```python
from build123d import *

# Parameters (mm, degrees)
BOSS_EXTRUDE1_DEPTH = 30
SHELL1_T            = 3


with BuildPart() as part:
    # Sketch1 → Boss-Extrude1 (new body)
    with BuildSketch(Plane(origin=(0, 0, 0), x_dir=(1, 0, 0), z_dir=(0, 1, 0))):
        Polygon((20.5, 48.994047619), (-20.5, 48.994047619), (-20.5, -1.005952381), (-50, -1.005952381), (-50, -51.005952381), (50, -51.005952381), (50, -1.005952381), (20.5, -1.005952381), align=None)
    extrude(amount=BOSS_EXTRUDE1_DEPTH)

    # Shell1
    shell1_openings = [part.faces().sort_by_distance(p)[0] for p in [
        (0, 30, 11.466945289),
    ]]
    offset(amount=SHELL1_T, openings=shell1_openings, kind=Kind.INTERSECTION)


solid = part.part
```
The model under review builds one solid part; all positions refer to its coordinate system, in mm. A direction names the side the tool comes from. Coordinates: 2 decimals unless noted, no trailing zeros. Write each loop counter-clockwise with the first axis right and the second up, starting at its lowest first coordinate (ties: lowest second). Pieces come first, ordered by that corner, then holes.
1) We need section B-B on x = -17. State the section outline as (y, z) points.
2) Machinability: for faces 1 (the face through (-50, 15, 26)), 2 (the face through (23.5, 13, -27)), 3 (the face through (-38, 13, -1.994)), which of the approach directions +Z, -Z, +X, -X, +Y, -Y give a long, thin tool a straight path to every point of the face, cutting with its end or side? Answer none if there is none.
3) We need section A-A on y = 6. State the section outline as (x, z) points, then the cut area to 3 significant figures.
4) To check wall thickness, follow probe 1 along X at (y, z) = (7, -47.5); probe 2 along X at (y, z) = (11, 19); probe 3 along Z at (x, y) = (-29, 6). State the ranges of each line that lie inside material, in increasing order.
5) Clearance check with flat-ended pins moving along their axes: pin 1 Ø6 at (x, z) = (13, 29) entering from +Y; pin 2 Ø12 at (y, z) = (9.5, -29) entering from +X; pin 3 Ø15 at (x, y) = (-34, 8.5) entering from -Z. State where each tip first meets the part, or that it passes through.
6) We need section C-C on z = 2.5. State the section outline as (x, y) points.
Answer list:
1. outline: (-3, -51.99) - (30, -51.99) - (30, -48.99) - (0, -48.99) - (0, 51.01) - (30, 51.01) - (30, 54.01) - (-3, 54.01) - close
2. face 1: +Y
2. face 2: -Z, +X, +Y, -Y
2. face 3: -Z, -X, +Y, -Y
3. outline: (-53, -1.99) - (-23.5, -1.99) - (-23.5, -51.99) - (23.5, -51.99) - (23.5, -1.99) - (53, -1.99) - (53, 54.01) - (-53, 54.01) - close; hole (-50, 1.01) - (-20.5, 1.01) - (-20.5, -48.99) - (20.5, -48.99) - (20.5, 1.01) - (50, 1.01) - (50, 51.01) - (-50, 51.01) - close
3. area: 1,240 mm2
4. probe 1: x = -23.5 to -20.5, 20.5 to 23.5
4. probe 2: x = -53 to -50, 50 to 53
4. probe 3: z = -1.99 to 1.01, 51.01 to 54.01
5. pin 1: stops at y = 0
5. pin 2: stops at x = 23.5
5. pin 3: stops at z = -1.99
6. outline: (-53, -3) - (53, -3) - (53, 30) - (50, 30) - (50, 0) - (-50, 0) - (-50, 30) - (-53, 30) - close
